Work out the finished part from the listing and answer in its coordinate system (mm). A direction names the side the tool comes from. Coordinates: 2 decimals unless noted, no trailing zeros. Write each loop counter-clockwise with the first axis right and the second up, starting at its lowest first coordinate (ties: lowest second). Pieces come first, ordered by that corner, then holes. Notation, with made-up numbers: (-37.75, -12.75) - (12.25, -12.75) arc R12 cw to (12.25, -6.75) - close; hole circle Ø11 at (-34.5, -2). An arc over 180 degrees is marked (long way). Answer as a JSON object with one key per item and string values. Group by question number.
from build123d import *

# Parameters (mm, degrees)
SKETCH_1_R          = 25
EXTRUDE_1_DEPTH     = 42.5
EXTRUDE_1_2_DEPTH   = 42.5
SKETCH_2_R          = 25
SKETCH_2_R_2        = 19
CUT_EXTRUDE_1_DEPTH = 10
CHAMFER_1_SIZE      = 2
SKETCH_3_R          = 5
EXTRUDE_2_DEPTH     = 8
SKETCH_4_W          = 100
SKETCH_4_H          = 359
EXTRUDE_3_DEPTH     = 8
CHAMFER_2_SIZE      = 3
EXTRUDE_START       = 22
SKETCH_5_R          = 19
EXTRUDE_4_DEPTH     = 22
SKETCH_7_R          = 12.691244745
CUT_EXTRUDE_2_DEPTH = 10
SKETCH_8_R          = 19
EXTRUDE_5_DEPTH     = 20
EXTRUDE_6_DEPTH     = 20
CHAMFER_3_SIZE      = 2
CHAMFER_4_SIZE      = 2
SKETCH_11_R         = 27
EXTRUDE_8_DEPTH     = 2


with BuildPart() as part:
    # Sketch 1 → Extrude 1 (new, symmetric)
    with BuildSketch(Plane.XY):
        with Locations((-27.5, 0)):
            Circle(SKETCH_1_R)
    extrude(amount=EXTRUDE_1_DEPTH, both=True)


with BuildPart() as body_2:
    # Sketch 1 → Extrude 1 2 (new, symmetric)
    with BuildSketch(Plane.XY):
        with Locations((27.5, 0)):
            Circle(SKETCH_1_R)
    extrude(amount=EXTRUDE_1_2_DEPTH, both=True)


with BuildPart() as cut_extrude_1_tool:
    # Sketch 2 → Cut-Extrude 1 (new, symmetric)
    # profile 1 of 2: a face of its own
    with BuildSketch(Plane.XY):
        with Locations((-27.5, 0)):
            Circle(SKETCH_2_R)
        with Locations((-27.5, 0)):
            Circle(SKETCH_2_R_2, mode=Mode.SUBTRACT)
    # profile 2 of 2: a face of its own
    with BuildSketch(Plane.XY):
        with Locations((27.5, 0)):
            Circle(SKETCH_2_R)
        with Locations((27.5, 0)):
            Circle(SKETCH_2_R_2, mode=Mode.SUBTRACT)
    extrude(amount=CUT_EXTRUDE_1_DEPTH, both=True)


with BuildPart() as part_1:
    add(part.part)

    # Cut-Extrude 1: cut by cut_extrude_1_tool
    add(cut_extrude_1_tool.part, mode=Mode.SUBTRACT)



with BuildPart() as body_2_1:
    add(body_2.part)

    # Cut-Extrude 1: cut by cut_extrude_1_tool
    add(cut_extrude_1_tool.part, mode=Mode.SUBTRACT)

    # Chamfer 1
    chamfer_1_edges = [body_2_1.edges().sort_by_distance(p)[0] for p in [
        (2.5, 0, -42.5),
        (2.5, 0, 42.5),
    ]]
    chamfer(chamfer_1_edges, length=CHAMFER_1_SIZE)


with BuildPart() as part_2:
    add(part_1.part)

    add(body_2_1.part)  # Extrude 2 merges body 2
    # Sketch 3 → Extrude 2 (add)
    with BuildSketch(Plane(origin=(0, 0, -42.5), x_dir=(-1, 0, 0), z_dir=(0, 0, -1))):
        with Locations(Location((-27.5, 0, 0), (0, 0, 180))):
            Circle(SKETCH_3_R)
        with Locations(Location((27.5, 0, 0), (0, 0, 180))):
            Circle(SKETCH_3_R)
    extrude_2 = extrude(amount=EXTRUDE_2_DEPTH)

    # Mirror 1: Extrude 2 across plane
    add(extrude_2.mirror(Plane.XY))

    # Sketch 4 → Extrude 3 (add)
    with BuildSketch(Plane(origin=(0, 0, -50.5), x_dir=(-1, 0, 0), z_dir=(0, 0, -1))):
        with Locations((0, 167.5)):
            Rectangle(SKETCH_4_W, SKETCH_4_H)
    extrude_3 = extrude(amount=EXTRUDE_3_DEPTH)

    # Mirror 2: Extrude 3 across plane
    add(extrude_3.mirror(Plane.XY))

    # Chamfer 2
    chamfer_2_edges = [part_2.edges().sort_by_distance(p)[0] for p in [
        (50, -12, -54.5),
        (-50, -12, -54.5),
        (50, -12, 54.5),
        (-50, -12, 54.5),
    ]]
    chamfer(chamfer_2_edges, length=CHAMFER_2_SIZE)

    # Sketch 5 → Extrude 4 (add)
    with BuildSketch(Plane(origin=(0, 0, -58.5), x_dir=(-1, 0, 0), z_dir=(0, 0, -1)).offset(EXTRUDE_START)):
        with Locations(Location((27.5, 0, 0), (0, 0, 180))):
            Circle(SKETCH_5_R)
        with Locations(Location((-27.5, 0, 0), (0, 0, 180))):
            Circle(SKETCH_5_R)
    extrude(amount=-EXTRUDE_4_DEPTH)

    # Sketch 7 → Cut-Extrude 2 (cut)
    with BuildSketch(Plane.XY.offset(-50.5)):
        with Locations((0, 284.128548052)):
            Circle(SKETCH_7_R)
    extrude(amount=-CUT_EXTRUDE_2_DEPTH, mode=Mode.SUBTRACT)

    # Sketch 8 → Extrude 5 (add)
    with BuildSketch(Plane(origin=(0, 0, -58.5), x_dir=(-1, 0, 0), z_dir=(0, 0, -1))):
        with Locations(Location((0, 284.128548052, 0), (0, 0, 180))):
            Circle(SKETCH_8_R)
    extrude(amount=EXTRUDE_5_DEPTH)

    # Sketch 9 → Extrude 6 (add)
    with BuildSketch(Plane(origin=(0, 0, -58.5), x_dir=(-1, 0, 0), z_dir=(0, 0, -1))):
        with BuildLine():
            Line((-47.663589703, 3.657187648), (-47.992568683, 0))
            ThreePointArc((-47.992568683, 0), (-41.99043428, -14.49043428), (-27.5, -20.492568683))
            Line((-27.5, -20.492568683), (-27.257396579, -20.491132589))
            Line((-27.257396579, -20.491132589), (27.5, -20.166995645))
            ThreePointArc((27.5, -20.166995645), (41.760219376, -14.260219376), (47.666995645, 0))
            Line((47.666995645, 0), (47.351318556, 3.554274177))
            Line((47.351318556, 3.554274177), (22.256216625, 286.105260405))
            ThreePointArc((22.256216625, 286.105260405), (0.012611737, 306.472370714), (-22.253970975, 286.130383715))
            Line((-22.253970975, 286.130383715), (-47.663589703, 3.657187648))
        make_face()
        with BuildLine():
            ThreePointArc((-19.514906453, 285.892832564), (-1.852338091, 303.635293483), (18.83403815, 289.534404199))
            Line((18.83403815, 289.534404199), (44.24481717, 3.429143794))
            ThreePointArc((44.24481717, 3.429143794), (40.523912674, -10.592577543), (27.5, -16.98253045))
            Line((27.5, -16.98253045), (-26.978378853, -17.781424905))
            ThreePointArc((-26.978378853, -17.781424905), (-27.239161385, -17.78716176), (-27.5, -17.789074183))
            ThreePointArc((-27.5, -17.789074183), (-41.187186564, -11.397239057), (-45.072256133, 3.200735692))
            Line((-45.072256133, 3.200735692), (-19.514906453, 285.892832564))
        make_face(mode=Mode.SUBTRACT)
    extrude(amount=EXTRUDE_6_DEPTH)

    # Chamfer 3
    chamfer_3_edges = [part_2.edges().sort_by_distance(p)[0] for p in [
        (-19, 284.128548052, -78.5),
        (-46.5, 0, -80.5),
        (8.5, 0, -80.5),
    ]]
    chamfer(chamfer_3_edges, length=CHAMFER_3_SIZE - 0.0001)  # a hair under: the kernel refuses the full size

    # Chamfer 4
    chamfer_4_edges = [part_2.edges().sort_by_distance(p)[0] for p in [
        (-52.5, 0, -42.5),
        (-52.5, 0, 42.5),
    ]]
    chamfer(chamfer_4_edges, length=CHAMFER_4_SIZE)

    # Sketch 11 → Extrude 8 (add)
    with BuildSketch(Plane(origin=(0, 0, -24.5), x_dir=(-1, 0, 0), z_dir=(0, 0, -1))):
        with Locations((27.5, 0)):
            Circle(SKETCH_11_R)
        with Locations((-27.5, 0)):
            Circle(SKETCH_11_R)
    extrude(amount=EXTRUDE_8_DEPTH)


solid = part_2.part
Q1. Section A-A on z = -65 is taken. Determine the outline of the cut face in (x, y).
Q2. For a pull along Z with two mould halves and no side action, classify faces 1 (the face through (27, 0, -80.5)), 2 (the face through (1, 347, 54)), 3 (the face through (2.524, 1.099, -17.148)) as +Z half, -Z half, draft (parallel to the pull), parting line (faces both ways), or undercut.
Q3. Consider L1, parallel to Z at x = 22.5, y = 12.5; L2, parallel to Z at x = -18, y = 200.5; L3, parallel to Y at x = 0, z = -53. Determine where each line is inside the solid, lowest interval first. Write a range as from..to.
Q4. Section B-B on y = 243.5 is taken. Determine the outline of the cut face in (x, z), plus the area to 3 significant figures.
Q5. Section C-C on z = 5.5 is taken. Determine the outline of the cut face in (x, y).
Q6. Flat-ended cylindrical pins translate along their axes: pin 1 Ø4 at (y, z) = (216.5, 56) entering from -X; pin 2 Ø9 at (x, z) = (16, 53) entering from -Y; pin 3 Ø10 at (y, z) = (220, -53) entering from +X. Find the tip coordinate at first contact, or state that the pin passes through.
Q7. A tool of negligible diameter and unlimited length cuts with its end or side. For faces 4 (the face through (42.15, -14.33, -68.36)), 5 (the face through (0, 284, -78.5)), 6 (the face through (2.524, 1.099, 25.464)), from which of +Z, -Z, +X, -X, +Y, -Y can it reach the whole face along a straight path? Write none if from no direction.
Numbers:
{
 "1": {"outline": "(-47.67, 0) arc R20.17 ccw to (-27.5, -20.17) - (27.5, -20.49) arc R20.49 ccw to (47.99, 0) - (22.25, 286.13) arc R22.34 ccw to (-22.26, 286.11) - close; circle Ø38 at (0, 284.13); hole (-43.66, 9.99) arc R19 cw (long way) to (-19.23, -17.1) - (20.56, -17.69) arc R19 cw (long way) to (44.62, 8.25) - (19.51, 285.89) arc R19.59 ccw to (-18.83, 289.53) - close"},
 "2": {"face 1": "-Z half", "face 2": "draft", "face 3": "undercut"},
 "3": {"L1": "z = -80.5..-50.5, -42.5..42.5, 50.5..58.5", "L2": "z = -58.5..-50.5, 50.5..58.5", "L3": "y = -12..271.44, 296.82..347"},
 "4": {"outline": "(-50, -58.5) - (-26.04, -58.5) - (-26.04, -78.5) - (-22.92, -78.5) - (-22.92, -58.5) - (23.35, -58.5) - (23.35, -78.5) - (26.09, -78.5) - (26.09, -58.5) - (50, -58.5) - (50, -50.5) - (-50, -50.5) - close; (-50, 50.5) - (50, 50.5) - (50, 58.5) - (-50, 58.5) - close", "area": "1,720 mm²"},
 "5": {"outline": "circle Ø38 at (-27.5, 0); circle Ø38 at (27.5, 0)"},
 "6": {"pin 1": "stops at x = -50", "pin 2": "stops at y = -12", "pin 3": "stops at x = 50"},
 "7": {"face 4": "-Z, +X, -Y", "face 5": "-Z, +X, -X, +Y", "face 6": "none"}
}
